from build123d import *

# Parameters (mm, degrees)
SKETCH_1_W      = 500
SKETCH_1_H      = 80
SKETCH_1_R      = 10
SKETCH_1_W_2    = 20
SKETCH_1_H_2    = 70
EXTRUDE_1_DEPTH = 30


with BuildPart() as part:
    # 草图1 → 凸台-拉伸1 (new body)
    # profile 1 of 3: a face of its own
    with BuildSketch(Plane.XY):
        Rectangle(SKETCH_1_W, SKETCH_1_H)
        Circle(SKETCH_1_R, mode=Mode.SUBTRACT)
    # profile 2 of 3: a face of its own
    with BuildSketch(Plane.XY):
        with Locations((-260, 0)):
            Rectangle(SKETCH_1_W_2, SKETCH_1_H_2)
    # profile 3 of 3: a face of its own
    with BuildSketch(Plane.XY):
        with Locations((260, 0)):
            Rectangle(SKETCH_1_W_2, SKETCH_1_H_2)
    extrude(amount=EXTRUDE_1_DEPTH)


solid = part.part
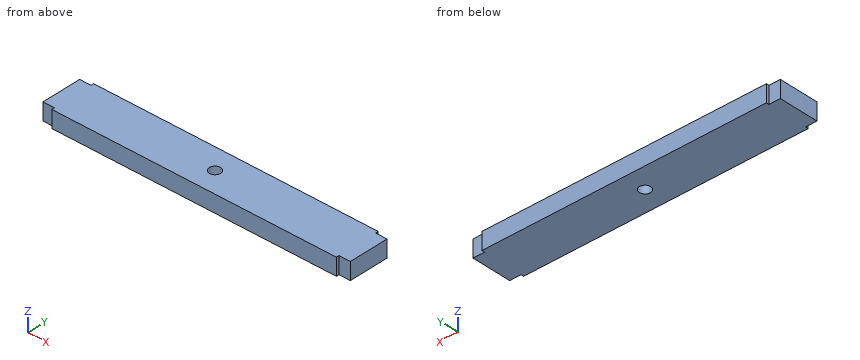
Build history of the part. All positions in model axes, mm. Round coordinates to 2 decimals unless told otherwise and drop trailing zeros. Loops run counter-clockwise (first coordinate to the right, second up) from the corner with the lowest first, then second, coordinate; pieces in that order, holes last. Notation, with made-up numbers: (71, -19.75) -> (102, -19.75) arc R17 ccw to (102, 2.25) -> close; hole circle Ø11 at (51, 56.25). An arc over 180 degrees is marked (long way). Use CSV: the item, a comma, the result in double quotes. Start each with the question number.
Q1. Saw through at C-C on y = 0. Give the cut face in (x, z).
Q2. Saw through at A-A on z = 11.25. Give the cut face in (x, y), and give its area (3 significant figures).
Q3. Saw through at B-B on x = 0. Give the cut face in (y, z).
Q4. Flat gauge pins, fed straight in: pin 1 Ø1.5 at (y, z) = (-38, 22) entering from -X; pin 2 Ø6 at (x, z) = (-263.5, 13) entering from -Y. Where does each tip first touch, or does it go through?
Q5. Drill centre lines: L1, parallel to Y at x = 0, z = 15.75; L2, parallel to X at y = 1, z = 24.5; L3, parallel to X at y = 5.5, z = 6. Where is each one in solid material? Low to high.
Solutions:
1,outline,"(-270, 0) -> (-10, 0) -> (-10, 30) -> (-270, 30) -> close; (10, 0) -> (270, 0) -> (270, 30) -> (10, 30) -> close"
2,outline,"(-270, -35) -> (-250, -35) -> (-250, -40) -> (250, -40) -> (250, -35) -> (270, -35) -> (270, 35) -> (250, 35) -> (250, 40) -> (-250, 40) -> (-250, 35) -> (-270, 35) -> close; hole circle Ø20 at (0, 0)"
2,area,"42,500 mm^2"
3,outline,"(-40, 0) -> (-10, 0) -> (-10, 30) -> (-40, 30) -> close; (10, 0) -> (40, 0) -> (40, 30) -> (10, 30) -> close"
4,pin 1,"stops at x = -250"
4,pin 2,"stops at y = -35"
5,L1,"y = -40 to -10, 10 to 40"
5,L2,"x = -270 to -9.95, 9.95 to 270"
5,L3,"x = -270 to -8.35, 8.35 to 270"
